from build123d import *

# Parameters (mm, degrees)
SKETCH1_W               = 45
SKETCH1_H               = 45
BOSS_EXTRUDE1_DEPTH     = 5.2
SKETCH2_W               = 9.7
SKETCH2_H               = 5.8
SKETCH2_W_2             = 5.8
SKETCH2_H_2             = 9.7
BOSS_EXTRUDE2_DEPTH     = 7
CUT_EXTRUDE1_DEPTH      = 35.078438931
CUT_EXTRUDE1_DEPTH_BACK = 35.078438931
SKETCH3_R               = 1.7
CUT_EXTRUDE2_DEPTH      = 2.5
FILLET1_R               = 2.5


with BuildPart() as part:
    # Sketch1 → Boss-Extrude1 (new body)
    with BuildSketch(Plane(origin=(0, 0, 0), x_dir=(1, 0, 0), z_dir=(0, 1, 0))):
        Rectangle(SKETCH1_W, SKETCH1_H)
    extrude(amount=-BOSS_EXTRUDE1_DEPTH)

    # Sketch2 → Boss-Extrude2 (add)
    with BuildSketch(Plane.XZ.offset(5.2)):
        with Locations((0, 14.9)):
            Rectangle(SKETCH2_W, SKETCH2_H)
        with Locations((-14.9, 0)):
            Rectangle(SKETCH2_W_2, SKETCH2_H_2)
        with Locations((14.9, 0)):
            Rectangle(SKETCH2_W_2, SKETCH2_H_2)
        with Locations((0, -14.9)):
            Rectangle(SKETCH2_W, SKETCH2_H)
    extrude(amount=BOSS_EXTRUDE2_DEPTH)

    # Sketch3 → Cut-Extrude1 (cut, two sides: drawn at the far end of the back side and taken through both)
    with BuildSketch(Plane(origin=(0, 0, 0), x_dir=(1, 0, 0), z_dir=(0, 1, 0)).offset(-CUT_EXTRUDE1_DEPTH_BACK)):
        with Locations(Location((-15.25, 15.25, 0), (0, 0, 270))):
            Circle(SKETCH3_R)
        with Locations(Location((15.25, 15.25, 0), (0, 0, 270))):
            Circle(SKETCH3_R)
        with Locations(Location((-15.25, -15.25, 0), (0, 0, 270))):
            Circle(SKETCH3_R)
        with Locations(Location((15.25, -15.25, 0), (0, 0, 270))):
            Circle(SKETCH3_R)
    extrude(amount=CUT_EXTRUDE1_DEPTH + CUT_EXTRUDE1_DEPTH_BACK, mode=Mode.SUBTRACT)

    # Sketch4 → Cut-Extrude2 (cut)
    with BuildSketch(Plane.XZ.offset(5.2)):
        Polygon((12.6, 13.720021787), (15.25, 12.190043573), (17.9, 13.720021787), (17.9, 16.779978213), (15.25, 18.309956427), (12.6, 16.779978213), align=None)
        Polygon((-13.720021787, 12.6), (-12.190043573, 15.25), (-13.720021787, 17.9), (-16.779978213, 17.9), (-18.309956427, 15.25), (-16.779978213, 12.6), align=None)
        Polygon((13.720021787, -12.6), (12.190043573, -15.25), (13.720021787, -17.9), (16.779978213, -17.9), (18.309956427, -15.25), (16.779978213, -12.6), align=None)
        Polygon((-12.6, -13.720021787), (-15.25, -12.190043573), (-17.9, -13.720021787), (-17.9, -16.779978213), (-15.25, -18.309956427), (-12.6, -16.779978213), align=None)
    extrude(amount=-CUT_EXTRUDE2_DEPTH, mode=Mode.SUBTRACT)

    # Fillet1
    fillet1_edges = [part.edges().sort_by_distance(p)[0] for p in [
        (22.5, -2.6, 22.5),
        (-22.5, -2.6, 22.5),
        (-22.5, -2.6, -22.5),
        (22.5, -2.6, -22.5),
    ]]
    fillet(fillet1_edges, radius=FILLET1_R)


solid = part.part
Design review of the part built by this model. Coordinates are the model's own, in mm. A direction names the side the tool comes from. Round coordinates to 2 decimals unless told otherwise and drop trailing zeros. Write each loop counter-clockwise with the first axis right and the second up, starting at its lowest first coordinate (ties: lowest second). Pieces come first, ordered by that corner, then holes. Notation, with made-up numbers: M 13.5,33.5 L 42.5,33.5 A29 ccw 42.5,70.5 Z; hole C 71,88.5 d3. An arc over 180 degrees is marked long. One line per item, written item: value. Start each with the question number.
1. Clearance check with flat-ended pins moving along their axes: P1, Ø1.5, axis at x = 6.5, z = -13, coming from the -Y side; P2, Ø6.5, axis at y = -7.5, z = 14, coming from the +X side; P3, Ø4, axis at x = 15.25, z = 15.25, coming from the -Y side; P4, Ø2, axis at y = -7.5, z = 0.5, coming from the +X side. State where each tip first meets the part, or that it passes through.
2. Take a section at D-D on x = -11. State the section outline as (y, z) points.
3. For faces 4 (the face through (4.85, -9, -15)), 5 (the face through (-17.8, -9, 0)), 6 (the face through (12.6, -4, 15)), list the 3-axis set-ups (+Z, -Z, +X, -X, +Y, -Y) from which the entire face can be reached by the end or side of a thin tool; tool diameter is ignored.
4. Draft analysis for pull direction X (two halves, no side actions). For faces 1 (the face through (15, -9, 4.85)), 2 (the face through (-12.6, -4, -15)), 3 (the face through (21.748, -2.636, -21.787)), state which applies: pulls with the +X half, pulls with the -X half, needs draft (parallel to the pull), parting line crosses it, or undercut.
5. Take a section at B-B on z = -1. State the section outline as (x, y) points, then the cut area to 3 significant figures.
6. To check wall thickness, follow probe 1 along Z at (x, y) = (-15.25, -0.95); probe 2 along Z at (x, y) = (-2, -10.75). State the ranges of each line that lie inside material, in increasing order. Write a range as from..to.
7. Take a section at A-A on y = -9.25. State the section outline as (x, z) points.
8. Take a section at C-C on x = -2. State the section outline as (y, z) points.
Computed:
1. P1: stops at y = -5.2
1. P2: stops at x = 22.5
1. P3: stops at y = -2.7
1. P4: stops at x = 17.8
2. outline: M -5.2,-22.5 L 0,-22.5 L 0,22.5 L -5.2,22.5 Z
3. face 4: +Z, -Z, +X, -Y
3. face 5: +Z, -Z, -X, -Y
3. face 6: -Y
4. face 1: needs draft
4. face 2: undercut
4. face 3: pulls with the +X half
5. outline: M -22.5,-5.2 L -17.8,-5.2 L -17.8,-12.2 L -12,-12.2 L -12,-5.2 L 12,-5.2 L 12,-12.2 L 17.8,-12.2 L 17.8,-5.2 L 22.5,-5.2 L 22.5,0 L -22.5,0 Z
5. area: 315 mm²
6. probe 1: z = -22.5..-16.95, -13.55..13.55, 16.95..22.5
6. probe 2: z = -17.8..-12, 12..17.8
7. outline: M -17.8,-4.85 L -12,-4.85 L -12,4.85 L -17.8,4.85 Z; M -4.85,-17.8 L 4.85,-17.8 L 4.85,-12 L -4.85,-12 Z; M -4.85,12 L 4.85,12 L 4.85,17.8 L -4.85,17.8 Z; M 12,-4.85 L 17.8,-4.85 L 17.8,4.85 L 12,4.85 Z
8. outline: M -12.2,-17.8 L -5.2,-17.8 L -5.2,-22.5 L 0,-22.5 L 0,22.5 L -5.2,22.5 L -5.2,17.8 L -12.2,17.8 L -12.2,12 L -5.2,12 L -5.2,-12 L -12.2,-12 Z
